```python
from build123d import *

# Parameters (mm, degrees)
F0_R     = 12.5
F0_R_2   = 11.5
F1_DEPTH = 325
F3_D     = 6
F4_D     = 6


with BuildPart() as f1:
    # F0 (on Right) → F1 (new body)
    with BuildSketch(Plane.YZ):
        Circle(F0_R)
        Circle(F0_R_2, mode=Mode.SUBTRACT)
    extrude(amount=F1_DEPTH)

    # F3 (through all)
    with Locations(Plane(origin=(0, 0, 0), x_dir=(1, 0, 0), z_dir=(0, 0, -1))):
        with Locations((20, 0)):
            Hole(F3_D / 2)

    # F4 (through all)
    with Locations(Plane.XY):
        with Locations((20, 0)):
            Hole(F4_D / 2)


solid = f1.part
```
The model under review builds one solid part; all positions refer to its coordinate system, in mm. Give positions to 0.01 mm unless a question says otherwise; leave off trailing zeros. Write each loop counter-clockwise with the first axis right and the second up, starting at its lowest first coordinate (ties: lowest second). Pieces come first, ordered by that corner, then holes. Notation, with made-up numbers: M -7,65.5 L 49,65.5 A12 ccw 49,81.5 Z; hole C -19,28 d10. An arc over 180 degrees is marked long. Answer in a Markdown table with one row per item.
Item 1: For P1, Ø14, axis at y = 0, z = 0, coming from the -X side; P2, Ø1, axis at x = 44, z = 9, coming from the -Y side; P3, Ø6, axis at x = 69.5, y = -7, coming from the -Z side; P4, Ø1.5, axis at x = 286, z = -3, coming from the -Y side, all flat-tipped, find the tip position at first contact; note any pin that passes through.
Check sheet entries:
| item | result |
|---|---|
| P1 | through |
| P2 | y = -9.17 |
| P3 | z = -11.84 |
| P4 | y = -12.3 |
Item 2: Add section A-A on z = 0. Give the boundary of the cut face in (x, y), plus the area to 3 significant figures.
Check sheet entries:
| item | result |
|---|---|
| outline | M 0,-12.5 L 325,-12.5 L 325,-11.5 L 0,-11.5 Z; M 0,11.5 L 325,11.5 L 325,12.5 L 0,12.5 Z |
| area | 650 mm2 |
Item 3: Draft analysis for pull direction X (two halves, no side actions). For faces 1 (the face through (160.2, -1.5, 11.4)), 2 (the face through (18.39, -2.53, 11.81)), 3 (the face through (0, 11, -4)), state which applies: +X half, -X half, draft (parallel to the pull), parting line (faces both ways), or undercut.
Check sheet entries:
| item | result |
|---|---|
| face 1 | draft |
| face 2 | undercut |
| face 3 | -X half |
Item 4: For line 1 along Z through (x, y) = (85, 0); line 2 along Z through (x, y) = (239.5, 6.75); line 3 along Y through (x, z) = (117.5, -9.25), list the stretches that pass through material, from the lowest coordinate up.
Check sheet entries:
| item | result |
|---|---|
| line 1 | -12.5 to -11.5, 11.5 to 12.5 |
| line 2 | -10.52 to -9.31, 9.31 to 10.52 |
| line 3 | -8.41 to -6.83, 6.83 to 8.41 |
Item 5: Add section C-C on x = 112. Give the boundary of the cut face in (y, z).
Check sheet entries:
| item | result |
|---|---|
| outline | C 0,0 d25; hole C 0,0 d23 |
Item 6: Add section B-B on y = -7.5. Give the boundary of the cut face in (x, z), plus the area to 3 significant figures.
Check sheet entries:
| item | result |
|---|---|
| outline | M 0,-10 L 325,-10 L 325,-8.72 L 0,-8.72 Z; M 0,8.72 L 325,8.72 L 325,10 L 0,10 Z |
| area | 833 mm2 |
